Build history of the part. All positions in model axes, mm. A direction names the side the tool comes from. Coordinates: 2 decimals unless noted, no trailing zeros. Loops run counter-clockwise (first coordinate to the right, second up) from the corner with the lowest first, then second, coordinate; pieces in that order, holes last.
(1) Flat gauge pins, fed straight in: P1, Ø1.5, axis at x = 3, z = -0.5, coming from the -Y side; P2, Ø1.8, axis at x = 0.5, z = -2, coming from the +Y side; P3, Ø1.8, axis at x = 0.5, z = -2, coming from the -Y side; P4, Ø2, axis at y = -3.5, z = 0.5, coming from the +X side. Where does each tip first touch, or does it go through?
(2) Slice it at B-B (x = -4). Give the cut face in (y, z), and give its area (3 significant figures).
(3) Wall check: L1, parallel to Z at x = 1.25, y = 5; L2, parallel to Z at x = -2, y = -5; L3, parallel to Y at x = -1.75, z = -2.3. Give the ranges that are in metal, low to high.
(4) Slice it at D-D (z = -2.1). Give the cut face in (x, y), and give its area (3 significant figures).
(5) Slice it at C-C (y = -6). Give the cut face in (x, z).
(6) Tool access for faces 1 (the face through (2.3, 1, -2)), 2 (the face through (-3.8, -6.5, 0.3)), 3 (the face through (0, 5.3, -2)), 4 (the face through (-2.3, 1, -2)): list every direction of +Z, -Z, +X, -X, +Y, -Y with a clear straight run to the whole face (end or side of a thin tool).
(7) Slice it at A-A (z = 0.55). Give the cut face in (x, y).
Autodesk Inventor part; units mm, degrees
ref_plane "YZ Plane" through (0, 0, 0) normal (1, 0, 0) x (0, 1, 0)
ref_plane "XZ Plane" through (0, 0, 0) normal (0, 1, 0) x (-1, 0, 0)
ref_plane "XY Plane" through (0, 0, 0) normal (0, 0, 1) x (1, 0, 0)
sketch "スケッチ1" plane through (0, 0, 0) normal (0, 0, 1) x (1, 0, 0)
  line L0 (-4.6, -6.5) -> (4.6, -6.5)
  line L1 (4.6, -6.5) -> (4.6, 6.5)
  line L2 (4.6, 6.5) -> (-4.6, 6.5)
  line L3 (-4.6, 6.5) -> (-4.6, -6.5)
  line L4 (-4.6, -6.5) -> (4.6, 6.5) construction
  line L5 (4.6, -6.5) -> (-4.6, 6.5) construction
  point P0 (0, 0)
  dimension "d0" = 9.2
  dimension "d1" = 13
extrude "押し出し1" add sketch "スケッチ1" along normal blind 0.2
sketch "スケッチ2" plane through (0, 0, 0.2) normal (0, 0, 1) x (1, 0, 0)
  line L0 (-4.6, -6.5) -> (-3.6, -6.5)
  line L1 (-3.6, -6.5) -> (-3.6, -5)
  line L2 (-3.6, -5) -> (-4.6, -5)
  line L3 (-4.6, -5) -> (-4.6, -6.5)
  line L4 (-4.6, -6.5) -> (4.6, -6.5)
  line L5 (4.6, -6.5) -> (3.6, -6.5)
  line L6 (3.6, -6.5) -> (3.6, -5)
  line L7 (3.6, -5) -> (4.6, -5)
  line L8 (4.6, -5) -> (4.6, -6.5)
  point P0 (0, 0)
  dimension "d4" = 1.5
  dimension "d5" = 1
extrude "押し出し2" add sketch "スケッチ2" along normal blind 0.7
sketch "スケッチ3" plane through (0, 0, 0) normal (0, 0, -1) x (-1, 0, 0)
  line L0 (-2.3, -2.9) -> (2.3, -2.9)
  line L1 (2.3, -2.9) -> (2.3, 5.3)
  line L2 (2.3, 5.3) -> (-2.3, 5.3)
  line L3 (-2.3, 5.3) -> (-2.3, -2.9)
  line L4 (-2.3, -2.9) -> (2.3, 5.3) construction
  line L5 (2.3, -2.9) -> (-2.3, 5.3) construction
  line L6 (-4.6, 6.5) -> (4.6, 6.5)
  point P0 (0, 0)
  point P1 (0, 1.2)
  point P2 (0, 1.2)
  dimension "d8" = 1.2
  dimension "d9" = 4.6
  dimension "d10" = 8.2
extrude "押し出し3" add sketch "スケッチ3" along normal blind 3.5
sketch "スケッチ4" plane through (0, 0, 0) normal (0, 0, -1) x (-1, 0, 0)
  line L0 (-1.6, -6.5) -> (1.6, -6.5)
  line L1 (1.6, -6.5) -> (1.6, -8.3)
  line L2 (1.6, -8.3) -> (-1.6, -8.3)
  line L3 (-1.6, -8.3) -> (-1.6, -6.5)
  line L4 (4.6, -6.5) -> (-4.6, -6.5)
  point P0 (0, 0)
  point P1 (0, -6.5)
  point P2 (0, -6.5)
  dimension "d13" = 3.2
  dimension "d14" = 1.8
extrude "押し出し4" add sketch "スケッチ4" against normal up to surface (0.2 mm away)
properties part number "terminal"
Response values:
1. P1: stops at y = -6.5
1. P2: stops at y = 5.3
1. P3: stops at y = -2.9
1. P4: stops at x = 4.6
2. outline: (-6.5, 0) - (6.5, 0) - (6.5, 0.2) - (-5, 0.2) - (-5, 0.9) - (-6.5, 0.9) - close
2. area: 3.65 mm2
3. L1: z = -3.5 to 0.2
3. L2: z = 0 to 0.2
3. L3: y = -2.9 to 5.3
4. outline: (-2.3, -2.9) - (2.3, -2.9) - (2.3, 5.3) - (-2.3, 5.3) - close
4. area: 37.7 mm2
5. outline: (-4.6, 0) - (4.6, 0) - (4.6, 0.9) - (3.6, 0.9) - (3.6, 0.2) - (-3.6, 0.2) - (-3.6, 0.9) - (-4.6, 0.9) - close
6. face 1: -Z, +X, +Y, -Y
6. face 2: +Z, -Z, -X, -Y
6. face 3: -Z, +X, -X, +Y
6. face 4: -Z, -X, +Y, -Y
7. outline: (-4.6, -6.5) - (-3.6, -6.5) - (-3.6, -5) - (-4.6, -5) - close; (3.6, -6.5) - (4.6, -6.5) - (4.6, -5) - (3.6, -5) - close
